```python
from build123d import *

# Parameters (mm, degrees)
F2_W         = 180
F2_H         = 180
F3_W         = 180
F3_H         = 180
F5_R         = 40
F6_T1_DEPTH  = 130
F6_S5_W      = 40
F6_S5_H      = 40
F6_T6_DEPTH  = 40
F6_S11_W     = 40
F6_S11_H     = 40
F6_T12_DEPTH = 40
F6_S17_W     = 40
F6_S17_H     = 40
F6_T18_DEPTH = 40
F6_S23_W     = 40
F6_S23_H     = 40
F6_T24_DEPTH = 40
F7_T         = 2.5
F0_R         = 2.5
F8_DEPTH     = 2.501


# Not quite as in the source:
# - a fillet or chamfer that OpenCascade refuses, or shapes differently, is made with other operations: its cross-section is extruded or revolved along the edge and cut away or added


with BuildPart() as f4:
    # F2 (on offset) → F4 section 0
    with BuildSketch(Plane.XY.offset(-70)):
        Rectangle(F2_W, F2_H)
    # F3 (on Top) → F4 section 1
    with BuildSketch(Plane.XY):
        Rectangle(F3_W, F3_H)
    loft()

    # F5
    f5_edges = [f4.edges().sort_by_distance(p)[0] for p in [
        (90, 0, 0),
        (0, -90, 0),
        (-90, 0, 0),
        (0, 90, 0),
    ]]
    fillet(f5_edges, radius=F5_R)

    # F6: fillet of radius 40 on 4 edges, made by hand

    # F6_s2 → F6_t1 (cut)
    with BuildSketch(Plane.XY.offset(-170)):
        with BuildLine():
            ThreePointArc((90, -50), (78.2842712475, -78.2842712475), (50, -90))
            Line((50, -90), (90, -90))
            Line((90, -90), (90, -50))
        make_face()
        with BuildLine():
            ThreePointArc((50, 90), (78.2842712475, 78.2842712475), (90, 50))
            Line((90, 50), (90, 90))
            Line((90, 90), (50, 90))
        make_face()
        with BuildLine():
            ThreePointArc((-50, 90), (-78.2842712475, 78.2842712475), (-90, 50))
            Line((-90, 50), (-90, 90))
            Line((-90, 90), (-50, 90))
        make_face()
        with BuildLine():
            ThreePointArc((-90, -50), (-78.2842712475, -78.2842712475), (-50, -90))
            Line((-50, -90), (-90, -90))
            Line((-90, -90), (-90, -50))
        make_face()
    extrude(amount=F6_T1_DEPTH, mode=Mode.SUBTRACT)


with BuildPart() as f6_tool4:
    # F6_s5 → F6_t6 (new body)
    with BuildSketch(Plane.YZ.offset(-50)):
        with Locations((-70, -20)):
            Rectangle(F6_S5_W, F6_S5_H)
    extrude(amount=-F6_T6_DEPTH)

    # F6_s7 → F6_t8 (revolve, cut)
    with BuildSketch(Plane(origin=(-50, -50, -40), x_dir=(0, 0.7071067812, -0.7071067812), z_dir=(0, 0.7071067812, 0.7071067812))):
        with BuildLine():
            ThreePointArc((0, -40), (40, 0), (0, 40))
            Line((0, 40), (0, -40))
        make_face()
    revolve(axis=Axis((-50, -50, -40), (-1, 0, 0)), mode=Mode.SUBTRACT)


with BuildPart() as f4_1:
    add(f4.part)

    # F6_t3: cut F6_tool4
    add(f6_tool4.part, mode=Mode.SUBTRACT)


with BuildPart() as f6_tool10:
    # F6_s11 → F6_t12 (new body)
    with BuildSketch(Plane.XZ.offset(-50)):
        with Locations((-70, -20)):
            Rectangle(F6_S11_W, F6_S11_H)
    extrude(amount=-F6_T12_DEPTH)

    # F6_s13 → F6_t14 (revolve, cut)
    with BuildSketch(Plane(origin=(-50, 50, -40), x_dir=(0.7071067812, 0, -0.7071067812), z_dir=(0.7071067812, 0, 0.7071067812))):
        with BuildLine():
            ThreePointArc((0, -40), (40, 0), (0, 40))
            Line((0, 40), (0, -40))
        make_face()
    revolve(axis=Axis((-50, 50, -40), (0, 1, 0)), mode=Mode.SUBTRACT)


with BuildPart() as f4_2:
    add(f4_1.part)

    # F6_t9: cut F6_tool10
    add(f6_tool10.part, mode=Mode.SUBTRACT)


with BuildPart() as f6_tool16:
    # F6_s17 → F6_t18 (new body)
    with BuildSketch(Plane.XZ.offset(-50)):
        with Locations((70, -20)):
            Rectangle(F6_S17_W, F6_S17_H)
    extrude(amount=-F6_T18_DEPTH)

    # F6_s19 → F6_t20 (revolve, cut)
    with BuildSketch(Plane(origin=(50, 50, -40), x_dir=(-0.7071067812, 0, -0.7071067812), z_dir=(0.7071067812, 0, -0.7071067812))):
        with BuildLine():
            ThreePointArc((0, -40), (40, 0), (0, 40))
            Line((0, 40), (0, -40))
        make_face()
    revolve(axis=Axis((50, 50, -40), (0, 1, 0)), mode=Mode.SUBTRACT)


with BuildPart() as f4_3:
    add(f4_2.part)

    # F6_t15: cut F6_tool16
    add(f6_tool16.part, mode=Mode.SUBTRACT)


with BuildPart() as f6_tool22:
    # F6_s23 → F6_t24 (new body)
    with BuildSketch(Plane.YZ.offset(50)):
        with Locations((-70, -20)):
            Rectangle(F6_S23_W, F6_S23_H)
    extrude(amount=F6_T24_DEPTH)

    # F6_s25 → F6_t26 (revolve, cut)
    with BuildSketch(Plane(origin=(50, -50, -40), x_dir=(0, 0.7071067812, -0.7071067812), z_dir=(0, -0.7071067812, -0.7071067812))):
        with BuildLine():
            ThreePointArc((0, -40), (40, 0), (0, 40))
            Line((0, 40), (0, -40))
        make_face()
    revolve(axis=Axis((50, -50, -40), (1, 0, 0)), mode=Mode.SUBTRACT)


with BuildPart() as f4_4:
    add(f4_3.part)

    # F6_t21: cut F6_tool22
    add(f6_tool22.part, mode=Mode.SUBTRACT)

    # F7
    f7_openings = [f4_4.faces().sort_by_distance(p)[0] for p in [
        (0, 0, -70),
    ]]
    offset(amount=F7_T, openings=f7_openings)

    # F0 (on Top) → F8 (cut, through all)
    with BuildSketch(Plane.XY):
        with BuildLine():
            Line((-10.4, 38.6243446546), (-2.6, 9.6560861637))
            ThreePointArc((-2.6, 9.6560861637), (0, 10), (2.6, 9.6560861637))
            Line((2.6, 9.6560861637), (10.4, 38.6243446546))
            ThreePointArc((10.4, 38.6243446546), (0, 40), (-10.4, 38.6243446546))
        make_face()
        with BuildLine():
            ThreePointArc((-9.6624159189, 2.576377032), (-8.6602540378, 5), (-7.0624159189, 7.0797091317))
            Line((-7.0624159189, 7.0797091317), (-28.2496636754, 28.3188365267))
            ThreePointArc((-28.2496636754, 28.3188365267), (-34.6410161514, 20), (-38.6496636754, 10.305508128))
            Line((-38.6496636754, 10.305508128), (-9.6624159189, 2.576377032))
        make_face()
        with BuildLine():
            ThreePointArc((-7.0624159189, -7.0797091317), (-8.6602540378, -5), (-9.6624159189, -2.576377032))
            Line((-9.6624159189, -2.576377032), (-38.6496636754, -10.305508128))
            ThreePointArc((-38.6496636754, -10.305508128), (-34.6410161514, -20), (-28.2496636754, -28.3188365267))
            Line((-28.2496636754, -28.3188365267), (-7.0624159189, -7.0797091317))
        make_face()
        with BuildLine():
            ThreePointArc((2.6, -9.6560861637), (0, -10), (-2.6, -9.6560861637))
            Line((-2.6, -9.6560861637), (-10.4, -38.6243446546))
            ThreePointArc((-10.4, -38.6243446546), (0, -40), (10.4, -38.6243446546))
            Line((10.4, -38.6243446546), (2.6, -9.6560861637))
        make_face()
        with BuildLine():
            ThreePointArc((9.6624159189, -2.576377032), (8.6602540378, -5), (7.0624159189, -7.0797091317))
            Line((7.0624159189, -7.0797091317), (28.2496636754, -28.3188365267))
            ThreePointArc((28.2496636754, -28.3188365267), (34.6410161514, -20), (38.6496636754, -10.305508128))
            Line((38.6496636754, -10.305508128), (9.6624159189, -2.576377032))
        make_face()
        with BuildLine():
            ThreePointArc((7.0624159189, 7.0797091317), (8.6602540378, 5), (9.6624159189, 2.576377032))
            Line((9.6624159189, 2.576377032), (38.6496636754, 10.305508128))
            ThreePointArc((38.6496636754, 10.305508128), (34.6410161514, 20), (28.2496636754, 28.3188365267))
            Line((28.2496636754, 28.3188365267), (7.0624159189, 7.0797091317))
        make_face()
        Circle(F0_R)
    extrude(amount=F8_DEPTH, mode=Mode.SUBTRACT)


solid = f4_4.part
```
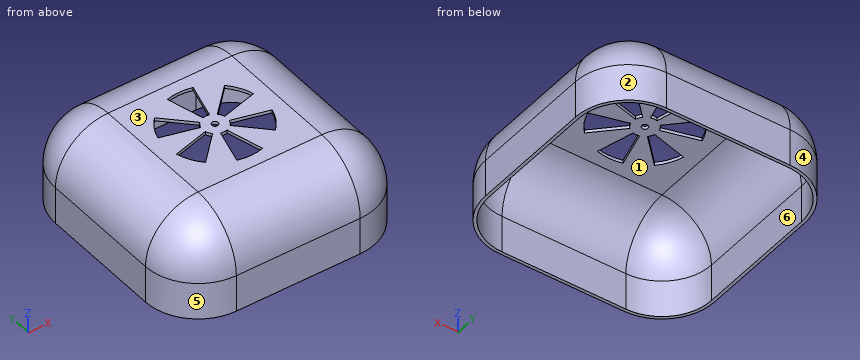
Build history of the part. All positions in model axes, mm. Face numbers are marked on the shaded views. A direction names the side the tool comes from. Give positions to 0.01 mm unless a question says otherwise; leave off trailing zeros. Loops run counter-clockwise (first coordinate to the right, second up) from the corner with the lowest first, then second, coordinate; pieces in that order, holes last. Notation, with made-up numbers: (51.25, 70) - (91.25, 70) arc R23 cw to (91.25, 98) - close; hole circle Ø1 at (-28.75, -2.5). An arc over 180 degrees is marked (long way). Use a Markdown table: item, result.
(1) Band-saw the part on D-D (x = 24). Give the cut face in (y, z).
Taken from the geometry:
| item | result |
|---|---|
| outline | (-92.5, -70) - (-90, -70) - (-90, -40) arc R40 cw to (-50, 0) - (-24.06, 0) - (-24.06, 2.5) - (-50, 2.5) arc R42.5 ccw to (-92.5, -40) - close; (-6.4, 0) - (6.4, 0) - (6.4, 2.5) - (-6.4, 2.5) - close; (24.06, 0) - (50, 0) arc R40 cw to (90, -40) - (90, -70) - (92.5, -70) - (92.5, -40) arc R42.5 ccw to (50, 2.5) - (24.06, 2.5) - close |
(2) Drop flat-ended pins along their axis: pin 1 Ø4 at (x, z) = (59.5, -8.5) entering from -Y; pin 2 Ø6 at (x, y) = (8.5, 45.5) entering from -Z; pin 3 Ø1.5 at (x, y) = (68.5, 1.5) entering from +Z. Give the stop position or say it passes through.
Taken from the geometry:
| item | result |
|---|---|
| pin 1 | y = -79.18 |
| pin 2 | z = 0 |
| pin 3 | z = -1.38 |
(3) Band-saw the part on B-B (z = -61). Give the cut face in (x, y).
Taken from the geometry:
| item | result |
|---|---|
| outline | (-92.5, -50) arc R42.5 ccw to (-50, -92.5) - (50, -92.5) arc R42.5 ccw to (92.5, -50) - (92.5, 50) arc R42.5 ccw to (50, 92.5) - (-50, 92.5) arc R42.5 ccw to (-92.5, 50) - close; hole (-90, -50) arc R40 ccw to (-50, -90) - (50, -90) arc R40 ccw to (90, -50) - (90, 50) arc R40 ccw to (50, 90) - (-50, 90) arc R40 ccw to (-90, 50) - close |
(4) Band-saw the part on A-A (y = 0). Give the cut face in (x, z).
Taken from the geometry:
| item | result |
|---|---|
| outline | (-92.5, -70) - (-90, -70) - (-90, -40) arc R40 cw to (-50, 0) - (-2.5, 0) - (-2.5, 2.5) - (-50, 2.5) arc R42.5 ccw to (-92.5, -40) - close; (2.5, 0) - (50, 0) arc R40 cw to (90, -40) - (90, -70) - (92.5, -70) - (92.5, -40) arc R42.5 ccw to (50, 2.5) - (2.5, 2.5) - close |
(5) Wall check: line 1 along X through (y, z) = (-38, -63); line 2 along Y through (x, z) = (55, -28). Give the ranges that are in metal, low to high.
Taken from the geometry:
| item | result |
|---|---|
| line 1 | -92.5 to -90, 90 to 92.5 |
| line 2 | -90.46 to -87.83, 87.83 to 90.46 |
(6) Band-saw the part on C-C (x = 0). Give the cut face in (y, z).
Taken from the geometry:
| item | result |
|---|---|
| outline | (-92.5, -70) - (-90, -70) - (-90, -40) arc R40 cw to (-50, 0) - (-40, 0) - (-40, 2.5) - (-50, 2.5) arc R42.5 ccw to (-92.5, -40) - close; (-10, 0) - (-2.5, 0) - (-2.5, 2.5) - (-10, 2.5) - close; (2.5, 0) - (10, 0) - (10, 2.5) - (2.5, 2.5) - close; (40, 0) - (50, 0) arc R40 cw to (90, -40) - (90, -70) - (92.5, -70) - (92.5, -40) arc R42.5 ccw to (50, 2.5) - (40, 2.5) - close |
(7) Pull direction X, two halves, no side cores. Call the marked faces 1, 2, 3 and 4: +X half, -X half, draft (parallel to the pull), parting line (faces both ways), or undercut.
Taken from the geometry:
| item | result |
|---|---|
| face 1 | undercut |
| face 2 | +X half |
| face 3 | draft |
| face 4 | -X half |
(8) Which spindle directions (+Z, -Z, +X, -X, +Y, -Y) get a long thin tool onto all of the face, cutting with end or side? Do the marked faces 5 and 6. Say none if no direction does.
Taken from the geometry:
| item | result |
|---|---|
| face 5 | +Z, -Z, -X, -Y |
| face 6 | -Z |
